The listing builds one solid part. Answer for the finished solid, in the listing's coordinates (mm). Face numbers are marked on the shaded views. A direction names the side the tool comes from. Round coordinates to 2 decimals unless told otherwise and drop trailing zeros. Order: outer loops, then holes, each group sorted by start corner. A loop starts at its lowest first (then second) coordinate and runs counter-clockwise, first axis right, second up. Notation, with made-up numbers: (59.25, 85.5) -> (107.25, 85.5) arc R17 cw to (107.25, 104.5) -> close; hole circle Ø4 at (47, -27.75). An arc over 180 degrees is marked (long way). Answer in a Markdown table with one row per item. Add a question column.
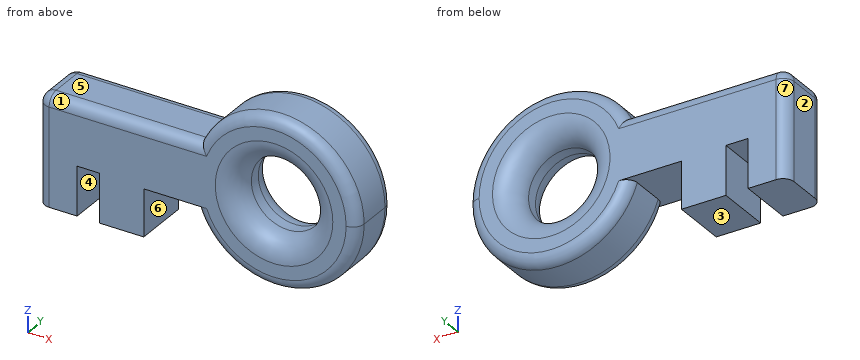
```python
from build123d import *

# Parameters (mm, degrees)
F0_R     = 3.299151
F1_DEPTH = 5
F2_R     = 1
F3_R     = 2
F4_R     = 2


with BuildPart() as f1:
    # F0 (on Front) → F1 (new body)
    with BuildSketch(Plane.XZ):
        with BuildLine():
            ThreePointArc((-10.135779, 4.245207), (-10.476368, 7.082065), (-9.731289, 9.840438))
            Line((-9.731289, 9.840438), (-24.275417, 9.840438))
            Line((-24.275417, 9.840438), (-24.275417, 0))
            Line((-24.275417, 0), (-20.750272, 0))
            Line((-20.750272, 0), (-20.750272, 4.406432))
            Line((-20.750272, 4.406432), (-18.750272, 4.406432))
            Line((-18.750272, 4.406432), (-18.750272, 0))
            Line((-18.750272, 0), (-14.741508, 0))
            Line((-14.741508, 0), (-14.741508, 4.245207))
            Line((-14.741508, 4.245207), (-10.135779, 4.245207))
        make_face()
        with BuildLine():
            ThreePointArc((-10.135779, 4.245207), (-1.833816, -0.868138), (4.50411, 6.541287))
            ThreePointArc((4.50411, 6.541287), (-1.302593, 13.847637), (-9.731289, 9.840438))
            ThreePointArc((-9.731289, 9.840438), (-10.476368, 7.082065), (-10.135779, 4.245207))
        make_face()
        with Locations((-2.99589, 6.541287)):
            Circle(F0_R, mode=Mode.SUBTRACT)
    extrude(amount=F1_DEPTH)

    # F2
    f2_edges = [f1.edges().sort_by_distance(p)[0] for p in [
        (-17.003353, -5, 9.840438),
        (-17.003353, 0, 9.840438),
        (-24.275417, 0, 4.920219),
        (-24.275417, -2.5, 9.840438),
        (-24.275417, -5, 4.920219),
        (-1.833816, -5, -0.868138),
        (-1.302593, -5, 13.847637),
        (-1.833816, 0, -0.868138),
        (-1.302593, 0, 13.847637),
    ]]
    fillet(f2_edges, radius=F2_R)

    # F3
    f3_edges = [f1.edges().sort_by_distance(p)[0] for p in [
        (-6.295041, 0, 6.541287),
    ]]
    fillet(f3_edges, radius=F3_R)

    # F4
    f4_edges = [f1.edges().sort_by_distance(p)[0] for p in [
        (-6.295041, -5, 6.541287),
    ]]
    fillet(f4_edges, radius=F4_R)


solid = f1.part
```
Item 1: The part is cut by section A-A, the plane x = -17. Give the vertices of the cut face in (y, z), and give its area (3 significant figures).
Item 2: For a pull along X with two mould halves and no side action, classify the marked faces 5, 6 and 7 as released by +X, released by -X, zero draft, split by the parting line, or undercut.
Item 3: The part is cut by section C-C, the plane x = -12.25. Give the vertices of the cut face in (y, z).
Item 4: Find the intervals of material crossed by probe 1 along X at (y, z) = (-4.15, 0.75); probe 2 along X at (y, z) = (-2.35, 0.75); probe 3 along X at (y, z) = (-2.35, 6.75), in increasing order. Write a range as [from, to].
Item 5: The part is cut by section B-B, the plane z = 0.5. State how many separate pieces and enclosed holes the cut face has, and give its area (3 significant figures).
Item 6: A tool of negligible diameter and unlimited length cuts with its end or side. For the marked faces 1, 2, 3 and 4, from which of +Z, -Z, +X, -X, +Y, -Y can it reach the whole face along a straight path? Write none if from no direction.
Item 7: Flat-ended cylindrical pins translate along their axes: P1, Ø2, axis at y = -1.5, z = 10, coming from the +X side; P2, Ø1.5, axis at x = -14.5, y = -2, coming from the +Z side; P3, Ø1.6, axis at x = -20, y = -2, coming from the -Z side. Find the tip coordinate at first contact, or state that the pin passes through.
Resolved:
| question | item | result |
|---|---|---|
| 1 | outline | (-5, 0) -> (0, 0) -> (0, 8.84) arc R1 ccw to (-1, 9.84) -> (-4, 9.84) arc R1 ccw to (-5, 8.84) -> close |
| 1 | area | 48.8 mm2 |
| 2 | face 5 | zero draft |
| 2 | face 6 | undercut |
| 2 | face 7 | released by -X |
| 3 | outline | (-5, 4.25) -> (0, 4.25) -> (0, 8.84) arc R1 ccw to (-1, 9.84) -> (-4, 9.84) arc R1 ccw to (-5, 8.84) -> close |
| 4 | probe 1 | [-24.26, -20.75], [-18.75, -14.74], [-7.74, 1.75] |
| 4 | probe 2 | [-24.28, -20.75], [-18.75, -14.74], [-7.76, 1.77] |
| 4 | probe 3 | [-24.28, -6.29], [0.3, 4.5] |
| 5 | separate pieces | 3 |
| 5 | enclosed holes | 0 |
| 5 | area | 80.1 mm2 |
| 6 | face 1 | +Z, -X, -Y |
| 6 | face 2 | +Z, -Z, -X, +Y, -Y |
| 6 | face 3 | -Z, -X, +Y, -Y |
| 6 | face 4 | -Z, +Y, -Y |
| 7 | P1 | x = 4.09 |
| 7 | P2 | z = 9.84 |
| 7 | P3 | z = 0 |
